Design review of the part shown in the three views and the two pictorial views. Dimensions are in mm from the part's minimum x, y and z. Round coordinates to 2 decimals unless told otherwise and drop trailing zeros. Loops run counter-clockwise (first coordinate to the right, second up) from the corner with the lowest first, then second, coordinate; pieces in that order, holes last. Notation, with made-up numbers: (-1, 66) -> (29, 66) arc R16 ccw to (29, 75) -> close; hole circle Ø2 at (-18.5, 20). An arc over 180 degrees is marked (long way). Write each question's results on one line, items separated by ' | '. Start each with the question number.
Item 1: For L1, parallel to Y at x = 180, z = 20.5; L2, parallel to X at y = 470, z = 22.75, list the stretches that pass through material, from the lowest coordinate up. Write a range as from..to.
Item 2: We need section C-C (z = 19). Give the boundary of the cut face in (x, y), and give its area (3 significant figures).
Item 3: We need section B-B (x = 172). Give the boundary of the cut face in (y, z).
Item 4: We need section A-A (y = 384.5). Give the boundary of the cut face in (x, z), and give its area (3 significant figures).
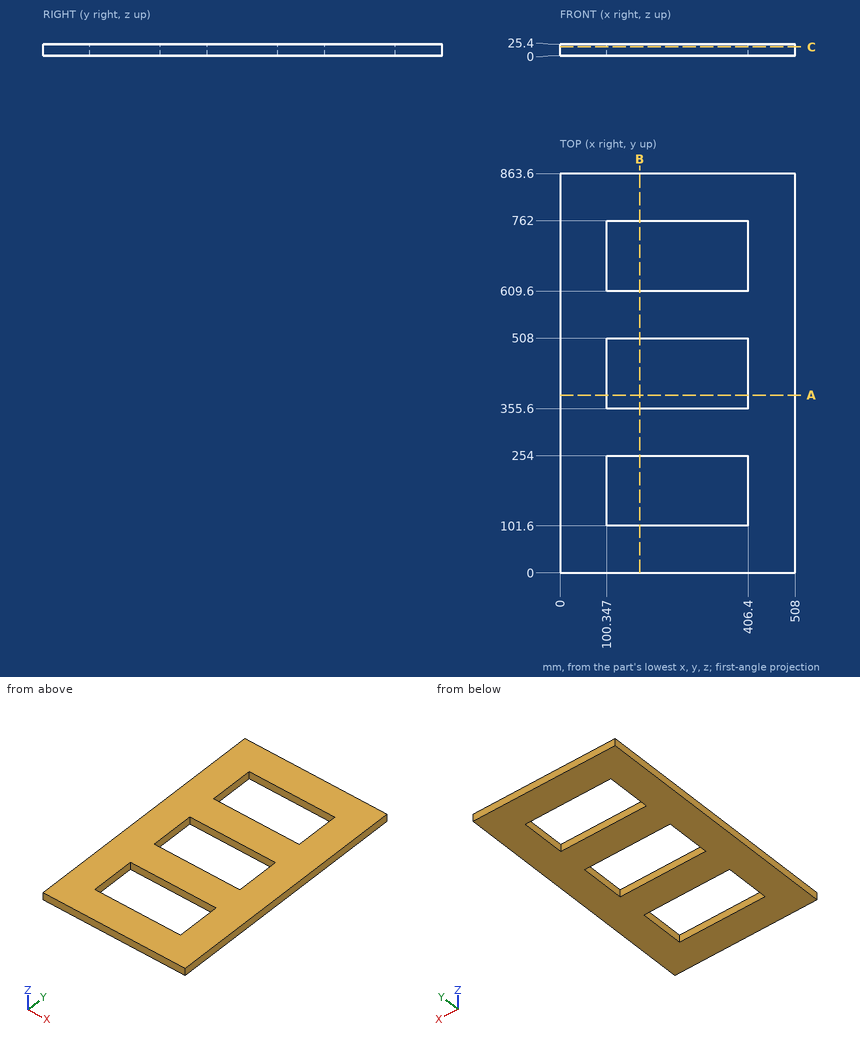
Here are the results:
1) L1: y = 0..101.6, 254..355.6, 508..609.6, 762..863.6 | L2: x = 0..100.35, 406.4..508
2) outline: (0, 0) -> (508, 0) -> (508, 863.6) -> (0, 863.6) -> close; hole (100.35, 101.6) -> (406.4, 101.6) -> (406.4, 254) -> (100.35, 254) -> close; hole (100.35, 355.6) -> (406.4, 355.6) -> (406.4, 508) -> (100.35, 508) -> close; hole (100.35, 609.6) -> (406.4, 609.6) -> (406.4, 762) -> (100.35, 762) -> close | area: 299,000 mm2
3) outline: (0, 0) -> (101.6, 0) -> (101.6, 25.4) -> (0, 25.4) -> close; (254, 0) -> (355.6, 0) -> (355.6, 25.4) -> (254, 25.4) -> close; (508, 0) -> (609.6, 0) -> (609.6, 25.4) -> (508, 25.4) -> close; (762, 0) -> (863.6, 0) -> (863.6, 25.4) -> (762, 25.4) -> close
4) outline: (0, 0) -> (100.35, 0) -> (100.35, 25.4) -> (0, 25.4) -> close; (406.4, 0) -> (508, 0) -> (508, 25.4) -> (406.4, 25.4) -> close | area: 5,130 mm2
